Work out the finished part from the listing and answer in its coordinate system (mm). Face numbers are marked on the shaded views. A direction names the side the tool comes from. Round coordinates to 2 decimals unless told otherwise and drop trailing zeros. Write each loop counter-clockwise with the first axis right and the second up, starting at its lowest first coordinate (ties: lowest second). Pieces come first, ordered by that corner, then holes. Notation, with made-up numbers: (-38, 77) - (-24, 77) arc R28 ccw to (-24, 105) - close; hole circle Ø1 at (44, -28.75). An arc over 180 degrees is marked (long way). Answer as a JSON object with one key per item and string values.
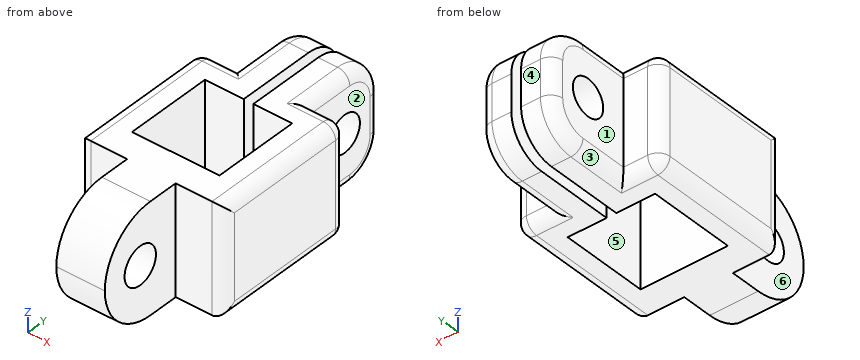
```python
from build123d import *

# Parameters (mm, degrees)
SKETCH_1_W          = 3
SKETCH_1_H          = 7
SKETCH_1_W_2        = 12
SKETCH_1_H_2        = 12
SKETCH_1_W_3        = 7
SKETCH_1_W_4        = 5
EXTRUDE_1_DEPTH     = 9
CUT_EXTRUDE_1_DEPTH = 17.911534525
FILLET_2_R          = 3
SKETCH_4_R          = 1.5
CUT_EXTRUDE_3_DEPTH = 19.193405399
FILLET_3_R          = 1
FILLET_4_R          = 1
FILLET_5_R          = 1
SKETCH_5_W          = 5
SKETCH_5_H          = 7
CUT_EXTRUDE_4_DEPTH = 9
EXTRUDE_2_DEPTH     = 7
FILLET_6_R          = 4.5
SKETCH_7_R          = 1.55
CUT_EXTRUDE_5_DEPTH = 4
SKETCH_8_W          = 3.1
SKETCH_8_H          = 0.1
CUT_EXTRUDE_6_DEPTH = 17.911534525


# Some blends are built 0.0001 mm under size
with BuildPart() as part:
    # 草图1 → 凸台-拉伸1 (new body)
    # profile 1 of 4: a face of its own
    with BuildSketch(Plane.XY):
        with Locations((-1.5, 9.5)):
            Rectangle(SKETCH_1_W, SKETCH_1_H)
    # profile 2 of 4: a face of its own
    with BuildSketch(Plane.XY):
        with Locations((1.5, 9.5)):
            Rectangle(SKETCH_1_W, SKETCH_1_H)
    # profile 3 of 4: a face of its own
    with BuildSketch(Plane.XY):
        Rectangle(SKETCH_1_W_2, SKETCH_1_H_2)
        Rectangle(SKETCH_1_W_3, SKETCH_1_H, mode=Mode.SUBTRACT)
    # profile 4 of 4: a face of its own
    with BuildSketch(Plane.XY):
        with Locations((1, -9.5)):
            Rectangle(SKETCH_1_W_4, SKETCH_1_H)
    extrude(amount=EXTRUDE_1_DEPTH)

    # 草图2 → 切除-拉伸1 (cut, through all)
    with BuildSketch(Plane.XY.offset(9)):
        Polygon((0, 13), (0.4, 13), (0.4, 3.5), (0, 3.5), (-0.4, 3.5), (-0.4, 13), align=None)
    extrude(amount=-CUT_EXTRUDE_1_DEPTH, mode=Mode.SUBTRACT)

    # 圆角2
    fillet_2_edges = [part.edges().sort_by_distance(p)[0] for p in [
        (1.7, 13, 9),
        (1.7, 13, 0),
        (-1.7, 13, 0),
        (-1.7, 13, 9),
    ]]
    fillet(fillet_2_edges, radius=FILLET_2_R)

    # 草图4 → 切除-拉伸3 (cut, through all)
    with BuildSketch(Plane(origin=(3, 0, 0), x_dir=(0, 0, -1), z_dir=(1, 0, 0))):
        with Locations((-4.5, 9.5)):
            Circle(SKETCH_4_R)
    extrude(amount=-CUT_EXTRUDE_3_DEPTH, mode=Mode.SUBTRACT)

    # 圆角3
    fillet_3_edges = [part.edges().sort_by_distance(p)[0] for p in [
        (3, 8, 9),
        (6, 0, 0),
        (3, 8, 0),
        (4.5, 6, 0),
        (6, 6, 4.5),
        (6, -6, 4.5),
        (4.5, 6, 9),
        (6, 0, 9),
        (3, 13, 4.5),
        (3, 12.121320344, 8.121320344),
        (3, 12.121320344, 0.878679656),
    ]]
    fillet(fillet_3_edges, radius=FILLET_3_R)

    # 圆角4
    fillet_4_edges = [part.edges().sort_by_distance(p)[0] for p in [
        (-3, 8, 9),
        (-6, 0, 0),
        (-4.5, 6, 0),
        (-3, 8, 0),
        (-4.5, 6, 9),
        (-6, 0, 9),
        (-6, -6, 4.5),
        (-3, 13, 4.5),
        (-3, 12.121320344, 8.121320344),
        (-3, 12.121320344, 0.878679656),
    ]]
    fillet(fillet_4_edges, radius=FILLET_4_R)

    # 圆角5
    # the kernel refuses this fillet: 1 mm, written as the material it takes off along each edge
    with BuildSketch(Plane(origin=(-5, 5, 8), x_dir=(0, 1, 0), z_dir=(-1, 0, 0))) as fillet_5_piece_1_section:
        Polygon((0, 0), (FILLET_5_R, 0), (FILLET_5_R, -FILLET_5_R), (0, -FILLET_5_R), align=None)
    fillet_5_piece_1 = extrude(amount=FILLET_5_R, mode=Mode.PRIVATE)
    fillet_5_piece_1 = fillet_5_piece_1 - Plane(origin=(-5, 5, 8), x_dir=(0, -0.7071067811865475, -0.7071067811865475), z_dir=(-1, 0, 0)) * Sphere(FILLET_5_R, mode=Mode.PRIVATE)
    add(fillet_5_piece_1, mode=Mode.SUBTRACT)
    with BuildSketch(Plane(origin=(-5, 5, 1), x_dir=(0, 1, 0), z_dir=(-1, 0, 0))) as fillet_5_piece_2_section:
        Polygon((0, 0), (FILLET_5_R, 0), (FILLET_5_R, FILLET_5_R), (0, FILLET_5_R), align=None)
    fillet_5_piece_2 = extrude(amount=FILLET_5_R, mode=Mode.PRIVATE)
    fillet_5_piece_2 = fillet_5_piece_2 - Plane(origin=(-5, 5, 1), x_dir=(0, -0.7071067811865475, 0.7071067811865475), z_dir=(-1, 0, 0)) * Sphere(FILLET_5_R, mode=Mode.PRIVATE)
    add(fillet_5_piece_2, mode=Mode.SUBTRACT)
    with BuildSketch(Plane(origin=(-6, 6, 1), x_dir=(0, -1, 0), z_dir=(0, 0, 1))) as fillet_5_piece_3:
        with BuildLine():
            CenterArc((FILLET_5_R, FILLET_5_R), FILLET_5_R, 180, 90)
            Line((0, FILLET_5_R), (0, 0))
            Line((0, 0), (FILLET_5_R, 0))
        make_face()
    extrude(amount=7, mode=Mode.SUBTRACT)

    # 草图5 → 切除-拉伸4 (cut)
    with BuildSketch(Plane.XY.offset(9)):
        with Locations((1, -9.5)):
            Rectangle(SKETCH_5_W, SKETCH_5_H)
    extrude(amount=-CUT_EXTRUDE_4_DEPTH, mode=Mode.SUBTRACT)

    # 草图6 → 凸台-拉伸2 (add)
    with BuildSketch(Plane.XZ.offset(6)):
        Polygon((0, 9), (-2, 9), (-2, 0), (0, 0), (2, 0), (2, 9), align=None)
    extrude(amount=EXTRUDE_2_DEPTH)

    # 圆角6
    fillet_6_edges = [part.edges().sort_by_distance(p)[0] for p in [
        (0, -13, 0),
        (0, -13, 9),
    ]]
    fillet(fillet_6_edges, radius=FILLET_6_R - 0.0001)  # a hair under: the kernel refuses the full size

    # 草图7 → 切除-拉伸5 (cut)
    with BuildSketch(Plane.ZY.offset(2)):
        with Locations((4.5, -9.5)):
            Circle(SKETCH_7_R)
    extrude(amount=-CUT_EXTRUDE_5_DEPTH, mode=Mode.SUBTRACT)

    # 草图8 → 切除-拉伸6 (cut, through all)
    with BuildSketch(Plane.XY.offset(9)):
        with Locations((-1.95, 3.55)):
            Rectangle(SKETCH_8_W, SKETCH_8_H)
        Polygon((0.4, 3.5), (3.5, 3.5), (3.6, 3.5), (3.6, 3.6), (0.4, 3.6), align=None)
        Polygon((3.6, 3.5), (3.5, 3.5), (3.5, -3.5), (3.5, -3.6), (3.6, -3.6), align=None)
        Polygon((-3.6, -3.5), (-3.5, -3.5), (-3.5, 3.5), (-3.5, 3.6), (-3.6, 3.6), align=None)
        Polygon((3.5, -3.6), (3.5, -3.5), (-3.5, -3.5), (-3.6, -3.5), (-3.6, -3.6), align=None)
    extrude(amount=-CUT_EXTRUDE_6_DEPTH, mode=Mode.SUBTRACT)


solid = part.part
```
Item 1: Consider line 1 along Y through (x, z) = (-1.8, 4.5); line 2 along X through (y, z) = (5, 2.75); line 3 along X through (y, z) = (3.25, 1.25). Determine where each line is inside the solid, lowest interval first.
Results found:
{"line 1": "-13 to -11.05, -7.95 to -3.6, 3.6 to 8, 11 to 13", "line 2": "-6 to -0.4, 0.4 to 6", "line 3": "-6 to -3.6, 3.6 to 6"}
Item 2: Determine the mould class of the marked faces 4, 5 and 6 for opening direction X: pulls with the +X half, pulls with the -X half, needs draft (parallel to the pull), parting line crosses it, or undercut.
Results found:
{"face 4": "needs draft", "face 5": "undercut", "face 6": "pulls with the -X half"}
Item 3: For the marked faces 1, 2 and 3, determine the directions among +Z, -Z, +X, -X, +Y, -Y from which every point of the face is accessible in a straight line to the end or side of a thin tool.
Results found:
{"face 1": "+Z, -Z, -X, +Y", "face 2": "+Z, -Z, +X, +Y", "face 3": "-Z, -X, +Y"}
Item 4: A cutting plane is placed at D-D (x = 3.25). Write down the section's boundary in (y, z), and give its area (3 significant figures).
Results found:
{"outline": "(-6, 0) - (-3.6, 0) - (-3.6, 9) - (-6, 9) - close; (3.6, 0) - (5, 0) arc R1 ccw to (6, 1) - (6, 8) arc R1 ccw to (5, 9) - (3.6, 9) - close", "area": "42.8 mm²"}
Item 5: Each of these flat-tipped pins is pushed along its axis until it touches: P1, Ø2, axis at y = -10, z = 5, coming from the -X side; P2, Ø2, axis at x = 4.5, z = 3.5, coming from the +Y side; P3, Ø2, axis at x = 4, z = 3, coming from the -Y side. Where does it stop, or does it pass through?
Results found:
{"P1": "x = -2", "P2": "y = 6", "P3": "y = -6"}
Item 6: A cutting plane is placed at A-A (x = -1.5). Give the number of separate pieces and of enclosed holes in the cut face, and give its area (3 significant figures).
Results found:
{"separate pieces": "2", "enclosed holes": "2", "area": "142 mm²"}
Item 7: A cutting plane is placed at C-C (y = 9.5). Write down the section's boundary in (x, z).
Results found:
{"outline": "(-3, 1) arc R1 ccw to (-2, 0) - (-0.4, 0) - (-0.4, 3) - (-3, 3) - close; (-3, 6) - (-0.4, 6) - (-0.4, 9) - (-2, 9) arc R1 ccw to (-3, 8) - close; (0.4, 0) - (2, 0) arc R1 ccw to (3, 1) - (3, 3) - (0.4, 3) - close; (0.4, 6) - (3, 6) - (3, 8) arc R1 ccw to (2, 9) - (0.4, 9) - close"}
Item 8: A cutting plane is placed at B-B (y = -2). Write down the section's boundary in (x, z), and give its area (3 significant figures).
Results found:
{"outline": "(-6, 1) arc R1 ccw to (-5, 0) - (-3.6, 0) - (-3.6, 9) - (-5, 9) arc R1 ccw to (-6, 8) - close; (3.6, 0) - (5, 0) arc R1 ccw to (6, 1) - (6, 8) arc R1 ccw to (5, 9) - (3.6, 9) - close", "area": "42.3 mm²"}
